Verification items for the finished model (mm, model axes). A direction names the side the tool comes from. Round coordinates to 2 decimals unless told otherwise and drop trailing zeros. Order: outer loops, then holes, each group sorted by start corner. A loop starts at its lowest first (then second) coordinate and runs counter-clockwise, first axis right, second up. Notation, with made-up numbers: M -30,78 L -8,78 A27 ccw -8,114 Z; hole C 16.5,51.25 d3. An arc over 180 degrees is marked long. Answer as a JSON object with one key per item and string values. Group by question number.
```python
from build123d import *

# Parameters (mm, degrees)
SKETCH_5_W          = 23.8
SKETCH_5_H          = 15.8
EXTRUDE_2_DEPTH     = 9.6
SKETCH_6_R          = 2.5
EXTRUDE_3_DEPTH     = 1.7
SKETCH_7_R          = 2.6
CUT_EXTRUDE_1_DEPTH = 1.8


with BuildPart() as part:
    # Эскиз5 → Бобышка-Вытянуть2 (new body)
    with BuildSketch(Plane(origin=(0, 0, 0), x_dir=(1, 0, 0), z_dir=(0, 1, 0))):
        with Locations((11.9, 7.9)):
            Rectangle(SKETCH_5_W, SKETCH_5_H)
    extrude(amount=EXTRUDE_2_DEPTH)

    # Эскиз6 → Бобышка-Вытянуть3 (add)
    with BuildSketch(Plane(origin=(0, 9.6, 0), x_dir=(1, 0, 0), z_dir=(0, 1, 0))):
        with Locations((3.9, 11.9)):
            Circle(SKETCH_6_R)
        with Locations((11.929146399, 11.9)):
            Circle(SKETCH_6_R)
        with Locations((19.958292799, 11.9)):
            Circle(SKETCH_6_R)
        with Locations((11.870853601, 3.9)):
            Circle(SKETCH_6_R)
        with Locations((19.9, 3.9)):
            Circle(SKETCH_6_R)
        with Locations((3.841707201, 3.9)):
            Circle(SKETCH_6_R)
    extrude(amount=EXTRUDE_3_DEPTH)

    # Эскиз7 → Вырез-Вытянуть1 (cut)
    with BuildSketch(Plane.XZ):
        with Locations((3.9, -3.9)):
            Circle(SKETCH_7_R)
        with Locations((11.9, -3.9)):
            Circle(SKETCH_7_R)
        with Locations((19.9, -3.9)):
            Circle(SKETCH_7_R)
        with Locations((11.9, -11.9)):
            Circle(SKETCH_7_R)
        with Locations((19.9, -11.9)):
            Circle(SKETCH_7_R)
        with Locations((3.9, -11.9)):
            Circle(SKETCH_7_R)
    extrude(amount=-CUT_EXTRUDE_1_DEPTH, mode=Mode.SUBTRACT)


solid = part.part
```
Q1. Tool access check on faces 5 (the face through (18.116, 10.438, -13.59)), 6 (the face through (12, 5, 0)), 7 (the face through (6.38, 0.89, -11.12)). Record the directions out of +Z, -Z, +X, -X, +Y, -Y that give a thin tool (end or side, any length) a straight path to the whole face; none if there is none.
Q2. Cross-section at B-B, the plane x = 12.25. Record the cut outline in (y, z), then the cut area to 3 significant figures.
Q3. Thickness scan on line 1 (Z direction, x = 11.9, y = 1.2); line 2 (Y direction, x = 5.75, z = -2.25); line 3 (Y direction, x = 19, z = -7.5). Record the ranges inside material, lowest first. Write a range as from..to.
Q4. Cross-section at C-C, the plane x = 20.75. Record the cut outline in (y, z), then the cut area to 3 significant figures.
Q5. Release check for a two-part mould opening along X. For faces 1 (the face through (12, 1.8, -4)), 2 (the face through (12, 0, -8)), 3 (the face through (23.8, 5, -8)), 4 (the face through (9.373, 10.438, -4.01)) record: released by +X, released by -X, zero draft, split by the parting line, or undercut.
Q6. Cross-section at A-A, the plane z = -3.9. Record the cut outline in (x, y), then the cut area to 3 significant figures.
Q7. Cross-section at D-D, the plane z = -7.5. Record the cut outline in (x, y), then the cut area to 3 significant figures.
Q8. Gauge pin test, flat end, axial feed: pin 1 Ø4.5 at (x, z) = (11.9, -3.9) entering from -Y. Record the tip position at first contact, or that the pin passes through.
Conclusion:
{
 "1": {"face 5": "+Y", "face 6": "+Z, +X, -X, +Y, -Y", "face 7": "-Y"},
 "2": {"outline": "M 0,-15.8 L 9.6,-15.8 L 9.6,-14.38 L 11.3,-14.38 L 11.3,-9.42 L 9.6,-9.42 L 9.6,-6.37 L 11.3,-6.37 L 11.3,-1.43 L 9.6,-1.43 L 9.6,0 L 0,0 L 0,-1.32 L 1.8,-1.32 L 1.8,-6.48 L 0,-6.48 L 0,-9.32 L 1.8,-9.32 L 1.8,-14.48 L 0,-14.48 Z", "area": "150 mm2"},
 "3": {"line 1": "-15.8..-14.5, -9.3..-6.5, -1.3..0", "line 2": "1.8..9.6", "line 3": "0..9.6"},
 "4": {"outline": "M 0,-15.8 L 9.6,-15.8 L 9.6,-14.27 L 11.3,-14.27 L 11.3,-9.53 L 9.6,-9.53 L 9.6,-6.25 L 11.3,-6.25 L 11.3,-1.55 L 9.6,-1.55 L 9.6,0 L 0,0 L 0,-1.44 L 1.8,-1.44 L 1.8,-6.36 L 0,-6.36 L 0,-9.44 L 1.8,-9.44 L 1.8,-14.36 L 0,-14.36 Z", "area": "150 mm2"},
 "5": {"face 1": "undercut", "face 2": "zero draft", "face 3": "released by +X", "face 4": "undercut"},
 "6": {"outline": "M 0,0 L 1.3,0 L 1.3,1.8 L 6.5,1.8 L 6.5,0 L 9.3,0 L 9.3,1.8 L 14.5,1.8 L 14.5,0 L 17.3,0 L 17.3,1.8 L 22.5,1.8 L 22.5,0 L 23.8,0 L 23.8,9.6 L 22.4,9.6 L 22.4,11.3 L 17.4,11.3 L 17.4,9.6 L 14.37,9.6 L 14.37,11.3 L 9.37,11.3 L 9.37,9.6 L 6.34,9.6 L 6.34,11.3 L 1.34,11.3 L 1.34,9.6 L 0,9.6 Z", "area": "226 mm2"},
 "7": {"outline": "M 0,0 L 23.8,0 L 23.8,9.6 L 0,9.6 Z", "area": "228 mm2"},
 "8": {"pin 1": "y = 1.8"}
}
